The listing builds one solid part. Answer for the finished solid, in the listing's coordinates (mm). A direction names the side the tool comes from. Coordinates: 2 decimals unless noted, no trailing zeros. Loops run counter-clockwise (first coordinate to the right, second up) from the corner with the lowest first, then second, coordinate; pieces in that order, holes last. Notation, with made-up numbers: M 54.25,78 L 88.25,78 A18 cw 88.25,113 Z; hole C 12.25,4 d9. An arc over 180 degrees is marked long. Return JSON: item names as keys, results as strings. Group by question number.
1. Section C-C (y = -0.5) is taken. Write down the section's boundary in (x, z), then the cut area to 3 significant figures.
2. Straight lines are drawn through the part: L1, parallel to X at y = -11.5, z = 1.45; L2, parallel to X at y = -9, z = 0.35; L3, parallel to Y at x = 25, z = 0.9. For each, find the intervals that lie inside material, in ascending order. Write a range as from..to.
3. The mould has two halves that part along X. Classify faces 6 (the face through (25.765, 2.312, 0.986)), 7 (the face through (-22.07, 6.15, 0.99)), 8 (the face through (-17.892, 13.325, 0.986)): pulls with the +X half, pulls with the -X half, needs draft (parallel to the pull), parting line crosses it, or undercut.
4. Given P1, Ø0.8, axis at y = -12, z = 1, coming from the +X side; P2, Ø1, axis at x = 14, z = 1, coming from the -Y side; P3, Ø0.5, axis at y = -12, z = 1, coming from the -X side; P4, Ø1, axis at x = -14, y = -7, coming from the -Z side, each flat-ended and moving along its own axis, determine where each tip first touches the part or whether it passes through.
5. Section B-B (x = 12) is taken. Write down the section's boundary in (y, z).
6. Which of the six approach directions +Z, -Z, +X, -X, +Y, -Y give full straight-line access (tool end or side, diameter ignored) to faces 1 (the face through (-25.79, -3.13, 0.99)), 2 (the face through (-9.699, -13.215, 0.986)), 3 (the face through (25.64, -5.38, 0.99)), 4 (the face through (-26.5, -11, 1)), 5 (the face through (22.04, 6.14, 0.99))?
```python
from build123d import *

# Parameters (mm, degrees)
RESSALTO_EXTRUS_O1_DEPTH = 2


with BuildPart() as part:
    # Esboço1 → Ressalto-extrusão1 (new body)
    with BuildSketch(Plane.XY):
        with BuildLine():
            Line((-26.426946813, -7.319515656), (-24.880952381, -3.5))
            Line((-24.880952381, -3.5), (-26.734846007, -2.749614485))
            ThreePointArc((-26.734846007, -2.749614485), (-27.28040497, -2.212816705), (-27.286600063, -1.447474914))
            Line((-27.286600063, -1.447474914), (-24.285058001, 5.968099592))
            ThreePointArc((-24.285058001, 5.968099592), (-23.748260222, 6.513658555), (-22.98291843, 6.519853648))
            Line((-22.98291843, 6.519853648), (-21.129024804, 5.769468132))
            Line((-21.129024804, 5.769468132), (-18.252898169, 12.875192758))
            ThreePointArc((-18.252898169, 12.875192758), (-17.88488214, 13.329214314), (-17.325951356, 13.5))
            Line((-17.325951356, 13.5), (17.325951356, 13.5))
            ThreePointArc((17.325951356, 13.5), (17.88488214, 13.329214314), (18.252898169, 12.875192758))
            Line((18.252898169, 12.875192758), (21.129024804, 5.769468132))
            Line((21.129024804, 5.769468132), (22.98291843, 6.519853648))
            ThreePointArc((22.98291843, 6.519853648), (23.748260222, 6.513658555), (24.285058001, 5.968099592))
            Line((24.285058001, 5.968099592), (27.286600063, -1.447474914))
            ThreePointArc((27.286600063, -1.447474914), (27.28040497, -2.212816705), (26.734846007, -2.749614485))
            Line((26.734846007, -2.749614485), (24.880952381, -3.5))
            Line((24.880952381, -3.5), (26.426946813, -7.319515656))
            ThreePointArc((26.426946813, -7.319515656), (26.481566812, -7.503589097), (26.5, -7.694708414))
            Line((26.5, -7.694708414), (26.5, -13.5))
            Line((26.5, -13.5), (15, -13.5))
            ThreePointArc((15, -13.5), (14.292893219, -13.207106781), (14, -12.5))
            Line((14, -12.5), (14, -11.5))
            ThreePointArc((14, -11.5), (12, -9.5), (10, -11.5))
            Line((10, -11.5), (10, -12.5))
            ThreePointArc((10, -12.5), (9.707106781, -13.207106781), (9, -13.5))
            Line((9, -13.5), (-9, -13.5))
            ThreePointArc((-9, -13.5), (-9.707106781, -13.207106781), (-10, -12.5))
            Line((-10, -12.5), (-10, -11.5))
            ThreePointArc((-10, -11.5), (-12, -9.5), (-14, -11.5))
            Line((-14, -11.5), (-14, -12.5))
            ThreePointArc((-14, -12.5), (-14.292893219, -13.207106781), (-15, -13.5))
            Line((-15, -13.5), (-26.5, -13.5))
            Line((-26.5, -13.5), (-26.5, -7.694708414))
            ThreePointArc((-26.5, -7.694708414), (-26.481566812, -7.503589097), (-26.426946813, -7.319515656))
        make_face()
    extrude(amount=RESSALTO_EXTRUS_O1_DEPTH)


solid = part.part
```
Worked out:
{
 "1": {"outline": "M -26.9,0 L 26.9,0 L 26.9,2 L -26.9,2 Z", "area": "108 mm^2"},
 "2": {"L1": "-26.5..-14, -10..10, 14..26.5", "L2": "-26.5..26.5", "L3": "-13.5..-3.79, -3.45..4.2"},
 "3": {"face 6": "pulls with the +X half", "face 7": "undercut", "face 8": "pulls with the -X half"},
 "4": {"P1": "x = 26.5", "P2": "y = -13.37", "P3": "x = -26.5", "P4": "z = 0"},
 "5": {"outline": "M -9.5,0 L 13.5,0 L 13.5,2 L -9.5,2 Z"},
 "6": {"face 1": "+Z, -Z, -X", "face 2": "+Z, -Z, -Y", "face 3": "+Z, -Z, +X", "face 4": "+Z, -Z, -X, -Y", "face 5": "+Z, -Z, +Y"}
}
